```python
from build123d import *

# Parameters (mm, degrees)
SKETCH1_R           = 1.750000705
SKETCH1_R_2         = 2.000000004
BOSS_EXTRUDE1_DEPTH = 3
SKETCH4_R           = 3
SKETCH4_R_2         = 2
BOSS_EXTRUDE4_DEPTH = 1
SKETCH5_W           = 4
SKETCH5_H           = 100
EXTRUDE_THIN1_DEPTH = 2
CHAMFER1_SIZE       = 10


with BuildPart() as part:
    # Sketch1 → Boss-Extrude1 (new body)
    with BuildSketch(Plane.XY):
        with BuildLine():
            Line((-51.124108856, 36.963592514), (-41.497200727, 37.021376193))
            ThreePointArc((-41.497200727, 37.021376193), (-29.000000097, 43.850000709), (-16.502799466, 37.021376193))
            Line((-16.502799466, 37.021376193), (-6.715362892, 37.021376193))
            ThreePointArc((-6.715362892, 37.021376193), (-12.347919102, 45.842082936), (-21.231959071, 51.374206468))
            Line((-21.231959071, 51.374206468), (-21.231959071, 178.999762083))
            ThreePointArc((-21.231959071, 178.999762083), (-28.731959071, 186.499762083), (-36.231959071, 178.999762083))
            Line((-36.231959071, 178.999762083), (-36.231959071, 51.373953802))
            ThreePointArc((-36.231959071, 51.373953802), (-45.351125633, 45.897802101), (-51.124108856, 36.963592514))
        make_face()
        with Locations((-42.968060821, 43.288996652)):
            Circle(SKETCH1_R, mode=Mode.SUBTRACT)
        with Locations((-15.030000194, 43.288996652)):
            Circle(SKETCH1_R, mode=Mode.SUBTRACT)
        with Locations((-28.731959071, 178.999762083)):
            Circle(SKETCH1_R_2, mode=Mode.SUBTRACT)
    extrude(amount=BOSS_EXTRUDE1_DEPTH)

    # Sketch4 → Boss-Extrude4 (add)
    with BuildSketch(Plane.XY.offset(3)):
        with Locations(Location((-28.731959071, 178.999762083, 0), (0, 0, 180))):
            Circle(SKETCH4_R)
        with Locations((-28.731959071, 178.999762083)):
            Circle(SKETCH4_R_2, mode=Mode.SUBTRACT)
    extrude(amount=BOSS_EXTRUDE4_DEPTH)

    # Sketch5 → Extrude-Thin1 (add)
    with BuildSketch(Plane.XY.offset(3)):
        with Locations((-29.000000097, 114.00215714)):
            Rectangle(SKETCH5_W, SKETCH5_H)
    extrude(amount=EXTRUDE_THIN1_DEPTH)

    # Chamfer1
    # the kernel refuses this chamfer: 10 mm, written as the material it takes off along each edge
    with BuildSketch(Plane(origin=(-1.283170217, 164.00215714, 5), x_dir=(0, 0.0274958766105877, -0.9996219169112968), z_dir=(-1, 0, 0))) as chamfer1_piece_1_section:
        Polygon((CHAMFER1_SIZE * 0.999621916911, CHAMFER1_SIZE * 0.0274958766106), (-CHAMFER1_SIZE * 0.0274958766106, CHAMFER1_SIZE * 0.999621916911), (0, 0), align=None)
    chamfer1_piece_1 = extrude(amount=55.433659759, mode=Mode.PRIVATE)
    chamfer1_piece_1 = split(chamfer1_piece_1, bisect_by=Plane(origin=(-29.000000097, 159.483638622, 3), z_dir=(0, 0, 1)), keep=Keep.TOP, mode=Mode.PRIVATE)
    add(chamfer1_piece_1, mode=Mode.SUBTRACT)
    with BuildSketch(Plane(origin=(-56.716829977, 64.00215714, 5), x_dir=(0, -0.027495876610586317, -0.9996219169112968), z_dir=(1, 0, 0))) as chamfer1_piece_2_section:
        Polygon((CHAMFER1_SIZE * 0.999621916911, CHAMFER1_SIZE * 0.0274958766106), (-CHAMFER1_SIZE * 0.0274958766106, CHAMFER1_SIZE * 0.999621916911), (0, 0), align=None)
    chamfer1_piece_2 = extrude(amount=55.433659759, mode=Mode.PRIVATE)
    chamfer1_piece_2 = split(chamfer1_piece_2, bisect_by=Plane(origin=(-29.000000097, 68.520675659, 3), z_dir=(0, 0, 1)), keep=Keep.TOP, mode=Mode.PRIVATE)
    add(chamfer1_piece_2, mode=Mode.SUBTRACT)


solid = part.part
```
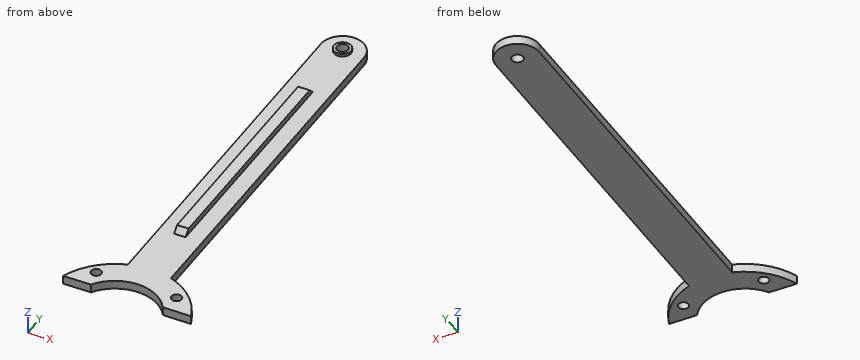
The model under review builds one solid part; all positions refer to its coordinate system, in mm. Round coordinates to 2 decimals unless told otherwise and drop trailing zeros. Write each loop counter-clockwise with the first axis right and the second up, starting at its lowest first coordinate (ties: lowest second). Pieces come first, ordered by that corner, then holes.
(1) We need section D-D on x = -47.5. Give the boundary of the cut face in (y, z), and give its area (3 significant figures).
(2) We need section B-B on x = -15.03. Give the boundary of the cut face in (y, z), and give its area (3 significant figures).
(3) We need section C-C on z = 1.65. Give the boundary of the cut face in (x, y).
(4) Insertion check: pin 1 (4.5 mm diameter, centred on x = -28.73, y = 179, fed in from +Z); pin 2 (0.9 mm diameter, centred on x = -13, z = 2, fed in from -Y); pin 3 (5 mm diameter, centred on x = -30, y = 95, fed in from -Z); pin 4 (2 mm diameter, centred on y = 129, z = 3.5, fed in from +X). Each pin has a flat end and moves straight along its axis. Give the tip position at first contact, or say it passes through.
(5) We need section A-A on y = 108. Give the boundary of the cut face in (x, z).
(6) Wall thickness on L1, parallel to Z at x = -35, y = 126; L2, parallel to X at y = 68.5, z = 1.35; L3, parallel to Y at x = -15.03, z = 1.4: over which ranges is each line inside the solid? List them lowest first.
Findings below:
1. outline: (36.99, 0) - (43.51, 0) - (43.51, 3) - (36.99, 3) - close
1. area: 19.6 mm2
2. outline: (37.02, 0) - (41.54, 0) - (41.54, 3) - (37.02, 3) - close; (45.04, 0) - (48.13, 0) - (48.13, 3) - (45.04, 3) - close
2. area: 22.8 mm2
3. outline: (-51.12, 36.96) - (-41.5, 37.02) arc R14.85 cw to (-16.5, 37.02) - (-6.72, 37.02) arc R23.68 ccw to (-21.23, 51.37) - (-21.23, 179) arc R7.5 ccw to (-36.23, 179) - (-36.23, 51.37) arc R23.51 ccw to start; hole circle Ø3.5 at (-42.97, 43.29); hole circle Ø4 at (-28.73, 179); hole circle Ø3.5 at (-15.03, 43.29)
4. pin 1: stops at z = 4
4. pin 2: stops at y = 37.02
4. pin 3: stops at z = 0
4. pin 4: stops at x = -21.23
5. outline: (-36.23, 0) - (-21.23, 0) - (-21.23, 3) - (-27, 3) - (-27, 5) - (-31, 5) - (-31, 3) - (-36.23, 3) - close
6. L1: z = 0 to 3
6. L2: x = -36.23 to -21.23
6. L3: y = 37.02 to 41.54, 45.04 to 48.13
